Model file for the job. Use its own axes, mm. A direction names the side the tool comes from. Coordinates: 2 decimals unless noted, no trailing zeros. Order: outer loops, then holes, each group sorted by start corner. A loop starts at its lowest first (then second) coordinate and runs counter-clockwise, first axis right, second up.
from build123d import *

# Parameters (mm, degrees)
F0_W     = 13.1121994928
F0_H     = 1.6037151217
F0_W_2   = 1.4255279675
F0_H_2   = 57.0257019255
F2_DEPTH = 2.5
F5_ANGLE = 180


with BuildPart() as f1:
    # F0 (on Front) → F1 (revolve)
    with BuildSketch(Plane.XZ):
        Polygon((-13.1121994928, 65.8466780561), (-13.1121994928, 67.4503931779), (-13.1121994928, 73.5088886696), (-16.3641842082, 73.5088886696), (-16.3641842082, 65.8466780562), (-15.271612443, 65.8466780562), (-13.8460844755, 65.8466780562), align=None)
        with Locations((-6.5560997464, 66.648535617)):
            Rectangle(F0_W, F0_H)
    revolve(axis=Axis((-8.1820921041, 0, 65.8466780562), (1, 0, 0)))

    # F0 (on Front) → F2 (join, symmetric)
    with BuildSketch(Plane.XZ):
        with Locations((-14.5588484593, 37.3338270934)):
            Rectangle(F0_W_2, F0_H_2)
    extrude(amount=F2_DEPTH, both=True)

    # F4 (on offset) → F5 (revolve)
    with BuildSketch(Plane(origin=(0, 0, 8.8209761307), x_dir=(1, 0, 0), z_dir=(0, 0, -1))):
        with BuildLine():
            Line((-14.5569266751, 2.5077068713), (-14.5569266751, 17.9110467434))
            add(Edge.make_bspline(
                [(-14.5569266751, 17.9110467434), (-21.6491705103, 17.9110467434), (-21.6491705103, 0), (-21.6491705103, -17.9110467434), (-14.5569266751, -17.9110467434)],
                knots=[3.1415926536, 3.1415926536, 3.1415926536, 4.7123889804, 4.7123889804, 6.2831853072, 6.2831853072, 6.2831853072], degree=2, weights=[1, 0.7071067812, 1, 0.7071067812, 1]))
            Line((-14.5569266751, -17.9110467434), (-14.5569266751, 2.5077068713))
        make_face()
    revolve(axis=Axis((-14.5569266751, 0, 8.8209761307), (0, -1, 0)), revolution_arc=F5_ANGLE)


solid = f1.part
Q1. Cut at C-C, the plane z = 22.5. List the corners of the cut face in (x, y), plus the area to 3 significant figures.
Established:
outline: (-15.27, -2.5) - (-13.85, -2.5) - (-13.85, 2.5) - (-15.27, 2.5) - close
area: 7.13 mm2
Q2. Cut at A-A, the plane x = -5.25. List the corners of the cut face in (y, z), plus the area to 3 significant figures.
Established:
outline: circle Ø3.21 at (0, 65.85)
area: 8.08 mm2
Q3. Mould opens along Z. For faces 4 (the face through (-15.272, 0, 33)), 5 (the face through (-15, -2.5, 34)), 6 (the face through (0, 0, 66)) say: pulls with the +Z half, pulls with the -Z half, needs draft (parallel to the pull), parting line crosses it, or undercut.
Established:
face 4: undercut
face 5: undercut
face 6: needs draft
Q4. Which spindle directions (+Z, -Z, +X, -X, +Y, -Y) get a long thin tool onto all of the face, cutting with end or side? Do faces 1 (the face through (-6.464, -0.071, 64.245)), 2 (the face through (-16.364, 0, 66)), 3 (the face through (-13.846, 0, 33)). Say none if no direction does.
Established:
face 1: +X
face 2: +Z, -X, +Y, -Y
face 3: +X, +Y, -Y
Q5. Drop flat-ended pins along their axis: P1, Ø12.5, axis at y = 1.5, z = 63.5, coming from the +X side; P2, Ø3, axis at x = -19.5, y = -6, coming from the +Z side; P3, Ø10, axis at y = -2.5, z = 14, coming from the +X side; P4, Ø7, axis at x = -15, y = -5, coming from the +Z side. Give the stop position or say it passes through.
Established:
P1: stops at x = 0
P2: stops at z = 8.82
P3: stops at x = -13.85
P4: stops at z = 73.36
Q6. Probe line 1 (X direction, y = 2, z = 60); line 2 (Z direction, x = -6.5, y = 0); line 3 (Z direction, x = -14.75, y = -5.5). List the from-to ranges inside material, lowest first.
Established:
line 1: x = -16.36 to -13.11
line 2: z = 64.24 to 67.45
line 3: z = 2.07 to 8.82, 60.51 to 71.18
Q7. Cut at B-B, the plane z = 59.5. List the corners of the cut face in (x, y).
Established:
outline: (-16.36, -4.29) - (-13.11, -4.29) - (-13.11, 4.29) - (-16.36, 4.29) - close
